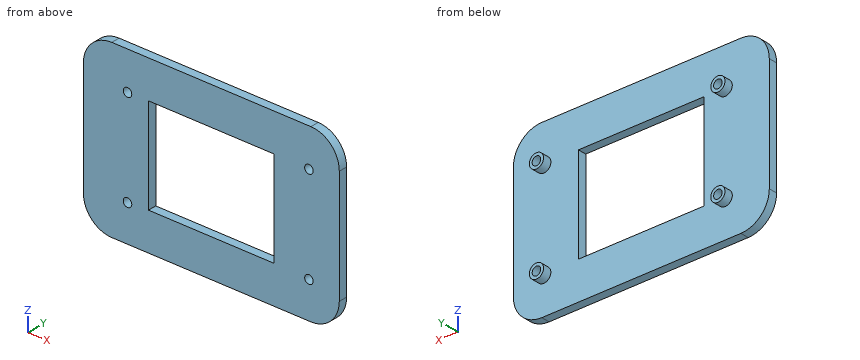
from build123d import *

# Parameters (mm, degrees)
SKETCH_1_W          = 90
SKETCH_1_H          = 60
EXTRUDE_1_DEPTH     = 3
SKETCH_2_R          = 1.5
SKETCH_2_W          = 44.23
SKETCH_2_H          = 33.59
CUT_EXTRUDE_1_DEPTH = 69.967825655
FILLET_1_R          = 10
SKETCH_3_R          = 2.5
EXTRUDE_2_DEPTH     = 3
SKETCH_4_R          = 1.5
CUT_EXTRUDE_2_DEPTH = 70.163292111


with BuildPart() as part:
    # 草圖1 → 填料-伸長1 (new body)
    with BuildSketch(Plane(origin=(0, 0, 0), x_dir=(1, 0, 0), z_dir=(0, 1, 0))):
        with Locations((-15.853658537, -2.317073171)):
            Rectangle(SKETCH_1_W, SKETCH_1_H)
    extrude(amount=EXTRUDE_1_DEPTH)

    # 草圖2 → 除料-伸長1 (cut, through all)
    with BuildSketch(Plane(origin=(0, 3, 0), x_dir=(1, 0, 0), z_dir=(0, 1, 0))):
        with Locations(Location((-45.338658537, 14.897926829, 0), (0, 0, 270))):
            Circle(SKETCH_2_R)
        with Locations(Location((-45.338658537, -18.972073171, 0), (0, 0, 270))):
            Circle(SKETCH_2_R)
        with Locations(Location((18.471341463, 14.897926829, 0), (0, 0, 270))):
            Circle(SKETCH_2_R)
        with Locations(Location((18.471341463, -18.972073171, 0), (0, 0, 270))):
            Circle(SKETCH_2_R)
        with Locations((-15.853658537, -2.317073171)):
            Rectangle(SKETCH_2_W, SKETCH_2_H)
    extrude(amount=-CUT_EXTRUDE_1_DEPTH, mode=Mode.SUBTRACT)

    # 圓角1
    fillet_1_edges = [part.edges().sort_by_distance(p)[0] for p in [
        (-60.853658537, 1.5, -27.682926829),
        (29.146341463, 1.5, -27.682926829),
        (29.146341463, 1.5, 32.317073171),
        (-60.853658537, 1.5, 32.317073171),
    ]]
    fillet(fillet_1_edges, radius=FILLET_1_R)

    # 草圖3 → 填料-伸長2 (add)
    with BuildSketch(Plane(origin=(0, 3, 0), x_dir=(1, 0, 0), z_dir=(0, 1, 0))):
        with Locations(Location((-45.338658537, 14.897926829, 0), (0, 0, 270))):
            Circle(SKETCH_3_R)
        with Locations(Location((-45.338658537, -18.972073171, 0), (0, 0, 270))):
            Circle(SKETCH_3_R)
        with Locations(Location((18.471341463, -18.972073171, 0), (0, 0, 270))):
            Circle(SKETCH_3_R)
        with Locations(Location((18.471341463, 14.897926829, 0), (0, 0, 270))):
            Circle(SKETCH_3_R)
    extrude(amount=EXTRUDE_2_DEPTH)

    # 草圖4 → 除料-伸長2 (cut, through all)
    with BuildSketch(Plane(origin=(0, 6, 0), x_dir=(1, 0, 0), z_dir=(0, 1, 0))):
        with Locations(Location((-45.338658537, 14.897926829, 0), (0, 0, 270))):
            Circle(SKETCH_4_R)
        with Locations(Location((-45.338658537, -18.972073171, 0), (0, 0, 270))):
            Circle(SKETCH_4_R)
        with Locations(Location((18.471341463, 14.897926829, 0), (0, 0, 270))):
            Circle(SKETCH_4_R)
        with Locations(Location((18.471341463, -18.972073171, 0), (0, 0, 270))):
            Circle(SKETCH_4_R)
    extrude(amount=-CUT_EXTRUDE_2_DEPTH, mode=Mode.SUBTRACT)


solid = part.part
Read the model definition and answer for the solid it produces. Units are mm, in the model's axes. Coordinates: 2 decimals unless noted, no trailing zeros. Loops run counter-clockwise (first coordinate to the right, second up) from the corner with the lowest first, then second, coordinate; pieces in that order, holes last. Notation, with made-up numbers: (-13.5, 70.25) -> (38.5, 70.25) arc R22 ccw to (38.5, 95.25) -> close; hole circle Ø11 at (89, 44.25). An arc over 180 degrees is marked (long way). Answer in a Markdown table with one row per item.
Item 1: A cutting plane is placed at C-C on y = 1.4. Determine the outline of the cut face in (x, z), plus the area to 3 significant figures.
Returned:
| item | result |
|---|---|
| outline | (-60.85, -17.68) arc R10 ccw to (-50.85, -27.68) -> (19.15, -27.68) arc R10 ccw to (29.15, -17.68) -> (29.15, 22.32) arc R10 ccw to (19.15, 32.32) -> (-50.85, 32.32) arc R10 ccw to (-60.85, 22.32) -> close; hole circle Ø3 at (-45.34, -14.9); hole circle Ø3 at (-45.34, 18.97); hole (-37.97, -14.48) -> (6.26, -14.48) -> (6.26, 19.11) -> (-37.97, 19.11) -> close; hole circle Ø3 at (18.47, -14.9); hole circle Ø3 at (18.47, 18.97) |
| area | 3,800 mm^2 |
Item 2: A cutting plane is placed at B-B on z = -5. Determine the outline of the cut face in (x, y).
Returned:
| item | result |
|---|---|
| outline | (-60.85, 0) -> (-37.97, 0) -> (-37.97, 3) -> (-60.85, 3) -> close; (6.26, 0) -> (29.15, 0) -> (29.15, 3) -> (6.26, 3) -> close |
Item 3: Each of these flat-tipped pins is pushed along its axis until it touches: P1, Ø1.8, axis at x = -45.34, z = 18.97, coming from the +Y side; P2, Ø6, axis at x = -20.5, z = 19.5, coming from the +Y side. Where does it stop, or does it pass through?
Returned:
| item | result |
|---|---|
| P1 | passes through |
| P2 | stops at y = 3 |
Item 4: Straight lines are drawn through the part: line 1 along X through (y, z) = (0.6, -15); line 2 along Z through (x, y) = (18.5, 1.85); line 3 along X through (y, z) = (1.85, 2). For each, find the intervals that lie inside material, in ascending order. Write a range as [from, to].
Returned:
| item | result |
|---|---|
| line 1 | x = [-60.85, -46.84], [-43.84, 16.97], [19.97, 29.15] |
| line 2 | z = [-27.68, -16.4], [-13.4, 17.47], [20.47, 32.32] |
| line 3 | x = [-60.85, -37.97], [6.26, 29.15] |
Item 5: A cutting plane is placed at D-D on x = 12.5. Determine the outline of the cut face in (y, z), plus the area to 3 significant figures.
Returned:
| item | result |
|---|---|
| outline | (0, -27.68) -> (3, -27.68) -> (3, 32.32) -> (0, 32.32) -> close |
| area | 180 mm^2 |
Item 6: A cutting plane is placed at A-A on x = -11.5. Determine the outline of the cut face in (y, z), plus the area to 3 significant figures.
Returned:
| item | result |
|---|---|
| outline | (0, -27.68) -> (3, -27.68) -> (3, -14.48) -> (0, -14.48) -> close; (0, 19.11) -> (3, 19.11) -> (3, 32.32) -> (0, 32.32) -> close |
| area | 79.2 mm^2 |
